Design review of the part shown in the three views and the two pictorial views. Dimensions are in mm from the part's minimum x, y and z. Coordinates: 2 decimals unless noted, no trailing zeros. Order: outer loops, then holes, each group sorted by start corner. A loop starts at its lowest first (then second) coordinate and runs counter-clockwise, first axis right, second up. Notation, with made-up numbers: (68.5, 11) - (85.5, 11) arc R21 cw to (85.5, 49) - close; hole circle Ø3 at (2.5, -11). An arc over 180 degrees is marked (long way). One line per item, written item: value. Start each with the question number.
(1) Consider section A-A on z = 2.5. Write out the cut boundary in (x, y) (1 decimal), then the cut area to 3 significant figures.
(2) To check wall thickness, follow line 1 along X through (y, z) = (80, 3.5); line 2 along X through (y, z) = (63, 4.75). State the ranges of each line that lie inside material, in increasing order.
(3) Clearance check with flat-ended pins moving along their axes: pin 1 (1.5 mm diameter, centred on y = 128, z = 4, fed in from -X); pin 2 (2 mm diameter, centred on y = 110, z = 4.5, fed in from +X); pin 3 (1 mm diameter, centred on x = 108, y = 41, fed in from -Z). State where each tip first meets the part, or that it passes through.
(4) Consider section B-B on y = 120.5. Write out the cut boundary in (x, z) (1 decimal).
(5) Consider section D-D on y = 55. Write out the cut boundary in (x, z).
(6) Consider section C-C on x = 16.5. Write out the cut boundary in (y, z), then the cut area to 3 significant figures.
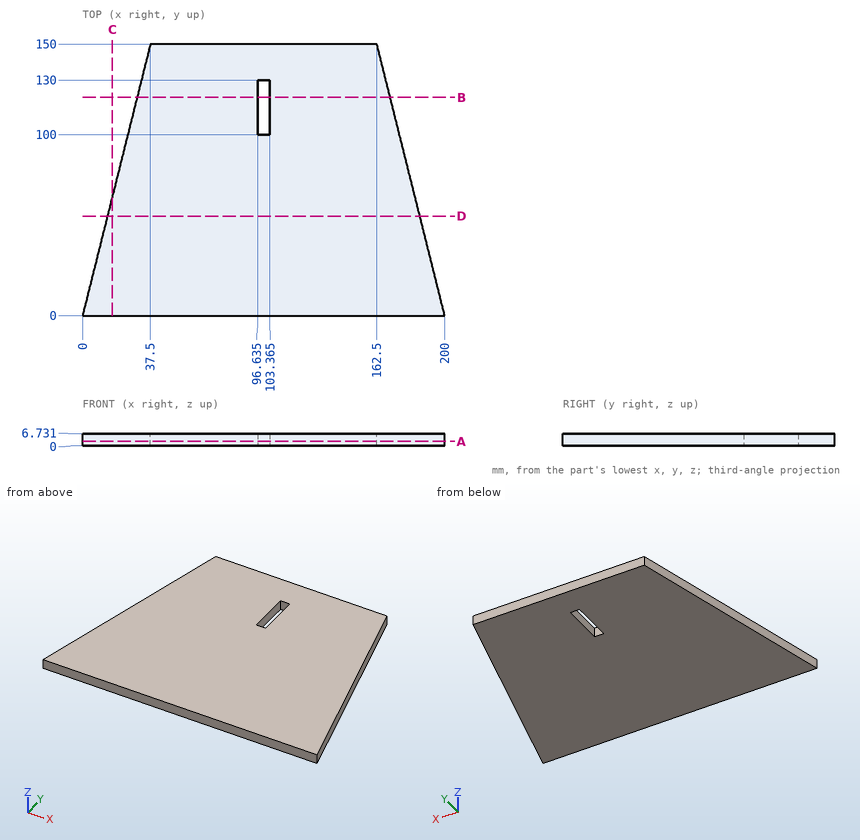
Geometry check:
1. outline: (0, 0) - (200, 0) - (162.5, 150) - (37.5, 150) - close; hole (96.6, 100) - (103.4, 100) - (103.4, 130) - (96.6, 130) - close
1. area: 24,200 mm^2
2. line 1: x = 20 to 180
2. line 2: x = 15.75 to 184.25
3. pin 1: stops at x = 31.81
3. pin 2: stops at x = 172.75
3. pin 3: stops at z = 0
4. outline: (30.1, 0) - (96.6, 0) - (96.6, 6.7) - (30.1, 6.7) - close; (103.4, 0) - (169.9, 0) - (169.9, 6.7) - (103.4, 6.7) - close
5. outline: (13.75, 0) - (186.25, 0) - (186.25, 6.73) - (13.75, 6.73) - close
6. outline: (0, 0) - (66, 0) - (66, 6.73) - (0, 6.73) - close
6. area: 444 mm^2
